from build123d import *

# Parameters (mm, degrees)
F0_R     = 9.5
F1_DEPTH = 1
F3_DEPTH = 10
F4_DEPTH = 35.9


with BuildPart() as f1:
    # F0 (on Front) → F1 (new body)
    with BuildSketch(Plane.XZ):
        with BuildLine():
            Line((25.5, 12.5), (-25.5, 12.5))
            ThreePointArc((-25.5, 12.5), (-26.914214, 11.914214), (-27.5, 10.5))
            Line((-27.5, 10.5), (-27.5, -10.5))
            ThreePointArc((-27.5, -10.5), (-26.914214, -11.914214), (-25.5, -12.5))
            Line((-25.5, -12.5), (25.5, -12.5))
            ThreePointArc((25.5, -12.5), (26.914214, -11.914214), (27.5, -10.5))
            Line((27.5, -10.5), (27.5, 10.5))
            ThreePointArc((27.5, 10.5), (26.914214, 11.914214), (25.5, 12.5))
        make_face()
        with Locations((-14.184796, 0)):
            Circle(F0_R, mode=Mode.SUBTRACT)
        with Locations((14.184796, 0)):
            Circle(F0_R, mode=Mode.SUBTRACT)
    extrude(amount=F1_DEPTH)

    # F0 (on Front) → F3 (join)
    with BuildSketch(Plane.XZ):
        with BuildLine():
            Line((25.5, 12.5), (-25.5, 12.5))
            ThreePointArc((-25.5, 12.5), (-26.914214, 11.914214), (-27.5, 10.5))
            Line((-27.5, 10.5), (-27.5, -10.5))
            ThreePointArc((-27.5, -10.5), (-26.914214, -11.914214), (-25.5, -12.5))
            Line((-25.5, -12.5), (25.5, -12.5))
            ThreePointArc((25.5, -12.5), (26.914214, -11.914214), (27.5, -10.5))
            Line((27.5, -10.5), (27.5, 10.5))
            ThreePointArc((27.5, 10.5), (26.914214, 11.914214), (25.5, 12.5))
        make_face()
        with Locations((-14.184796, 0)):
            Circle(F0_R, mode=Mode.SUBTRACT)
        with Locations((14.184796, 0)):
            Circle(F0_R, mode=Mode.SUBTRACT)
    extrude(amount=-F3_DEPTH)

    # F2 (on Front) → F4 (cut)
    with BuildSketch(Plane.XZ):
        with BuildLine():
            ThreePointArc((26.5, 10.5), (26.207107, 11.207107), (25.5, 11.5))
            Line((25.5, 11.5), (-25.5, 11.5))
            ThreePointArc((-25.5, 11.5), (-26.207107, 11.207107), (-26.5, 10.5))
            Line((-26.5, 10.5), (-26.5, -10.5))
            ThreePointArc((-26.5, -10.5), (-26.207107, -11.207107), (-25.5, -11.5))
            Line((-25.5, -11.5), (25.5, -11.5))
            ThreePointArc((25.5, -11.5), (26.207107, -11.207107), (26.5, -10.5))
            Line((26.5, -10.5), (26.5, 10.5))
        make_face()
    extrude(amount=-F4_DEPTH, mode=Mode.SUBTRACT)


solid = f1.part
Could you check a few things on this model? Use its own coordinates, in mm. A direction names the side the tool comes from. Coordinates: 2 decimals unless noted, no trailing zeros. Loops run counter-clockwise (first coordinate to the right, second up) from the corner with the lowest first, then second, coordinate; pieces in that order, holes last.
1. For faces 1 (the face through (-26.9, 4.42, 11.93)), 2 (the face through (-26.199, 4.93, 11.215)), which set-ups out of +Z, -Z, +X, -X, +Y, -Y let a thin tool reach every point of the face, with its end or its side?
2. Imagine slicing it at C-C (x = 10.5). Please give me the cut outline in (y, z).
3. Imagine slicing it at B-B (y = 4.5). Please give me the cut outline in (x, z), and give its area (3 significant figures).
4. We'd pull the mould along Z, two halves only. Please class faces 3 (the face through (26.9, 4.42, -11.93)), 4 (the face through (-21.724, -0.493, -5.781)), 5 (the face through (0, 4, 12.5)): released by +Z, released by -Z, zero draft, split by the parting line, or undercut.
5. Imagine slicing it at D-D (x = -1). Please give me the cut outline in (y, z), and give its area (3 significant figures).
6. For P1, Ø7, axis at x = 4.5, z = 1.5, coming from the +Y side; P2, Ø11.5, axis at x = 14.18, z = 0, coming from the +Y side, each with a flat end and sliding along its axis, tell me the tip position at first contact or that it passes through.
7. I need wall thicknesses on L1, parallel to Z at x = 24, y = 1.5; L2, parallel to X at y = 4.5, z = 0.5; L3, parallel to X at y = -0.5, z = 2.75. Which ranges of each line are inside material? Lowest first, please.
8. Imagine slicing it at A-A (z = 0). Please give me the cut outline in (x, y).
Computed values:
1. face 1: +Z, -X, +Y, -Y
1. face 2: +Y
2. outline: (-1, -12.5) - (10, -12.5) - (10, -11.5) - (0, -11.5) - (0, -8.76) - (-1, -8.76) - close; (-1, 8.76) - (0, 8.76) - (0, 11.5) - (10, 11.5) - (10, 12.5) - (-1, 12.5) - close
3. outline: (-27.5, -10.5) arc R2 ccw to (-25.5, -12.5) - (25.5, -12.5) arc R2 ccw to (27.5, -10.5) - (27.5, 10.5) arc R2 ccw to (25.5, 12.5) - (-25.5, 12.5) arc R2 ccw to (-27.5, 10.5) - close; hole (-26.5, -10.5) arc R1 ccw to (-25.5, -11.5) - (25.5, -11.5) arc R1 ccw to (26.5, -10.5) - (26.5, 10.5) arc R1 ccw to (25.5, 11.5) - (-25.5, 11.5) arc R1 ccw to (-26.5, 10.5) - close
3. area: 153 mm2
4. face 3: released by -Z
4. face 4: undercut
4. face 5: released by +Z
5. outline: (-1, -12.5) - (10, -12.5) - (10, -11.5) - (0, -11.5) - (0, 11.5) - (10, 11.5) - (10, 12.5) - (-1, 12.5) - close
5. area: 45.0 mm2
6. P1: stops at y = 0
6. P2: passes through
7. L1: z = -12.5 to -11.5, 11.5 to 12.5
7. L2: x = -27.5 to -26.5, 26.5 to 27.5
7. L3: x = -27.5 to -23.28, -5.09 to 5.09, 23.28 to 27.5
8. outline: (-27.5, -1) - (-23.68, -1) - (-23.68, 0) - (-26.5, 0) - (-26.5, 10) - (-27.5, 10) - close; (-4.68, -1) - (4.68, -1) - (4.68, 0) - (-4.68, 0) - close; (23.68, -1) - (27.5, -1) - (27.5, 10) - (26.5, 10) - (26.5, 0) - (23.68, 0) - close
